Build history of the part. All positions in model axes, mm. A direction names the side the tool comes from. Give positions to 0.01 mm unless a question says otherwise; leave off trailing zeros. Order: outer loops, then holes, each group sorted by start corner. A loop starts at its lowest first (then second) coordinate and runs counter-clockwise, first axis right, second up. Notation, with made-up numbers: (17, 79) - (57, 79) arc R28 cw to (57, 105) - close; hole circle Ø10 at (-25.75, -25.5). An arc over 180 degrees is marked (long way). Answer in a Markdown table with one row per item.
```python
from build123d import *

# Parameters (mm, degrees)
BOSS_EXTRU_1_DEPTH                                = 11.6
ESQUISSE2_R                                       = 10
BOSS_EXTRU_2_DEPTH                                = 3
ENL_V_MAT_EXTRU_1_DEPTH                           = 35.026203138
ENL_V_MAT_EXTRU_1_DEPTH_BACK                      = 35.026203138
ESQUISSE3_R                                       = 1.6
ESQUISSE3_R_2                                     = 3
CHAMBRAGE_POUR_VIS_SIX_PANS_CREUX_M41_D           = 3.2
CHAMBRAGE_POUR_VIS_SIX_PANS_CREUX_M41_CBORE_D     = 6
CHAMBRAGE_POUR_VIS_SIX_PANS_CREUX_M41_CBORE_DEPTH = 8
ENL_V_MAT_EXTRU_2_DEPTH                           = 38.537081666
ENL_V_MAT_EXTRU_2_DEPTH_BACK                      = 38.537081666
CHANFREIN1_SIZE                                   = 2
CHANFREIN2_SIZE                                   = 1


with BuildPart() as part:
    # Esquisse1 → Boss.-Extru.1 (new body)
    with BuildSketch(Plane(origin=(0, 0, 0), x_dir=(1, 0, 0), z_dir=(0, 1, 0))):
        Polygon((7.5, 27.85), (-7.5, 27.85), (-7.5, 10.85), (-13, 5), (-13, -5), (-7.5, -10.85), (-7.5, -27.85), (7.5, -27.85), (7.5, -10.85), (13, -5), (13, 5), (7.5, 10.85), align=None)
    extrude(amount=BOSS_EXTRU_1_DEPTH)

    # Esquisse2 → Boss.-Extru.2 (add)
    with BuildSketch(Plane(origin=(0, 11.6, 0), x_dir=(1, 0, 0), z_dir=(0, 1, 0))):
        with Locations(Location((0, 0, 0), (0, 0, 270))):
            Circle(ESQUISSE2_R)
    extrude(amount=BOSS_EXTRU_2_DEPTH)

    # Esquisse3 → Enlèv. mat.-Extru.1 (cut, two sides: drawn at the far end of the back side and taken through both)
    with BuildSketch(Plane.XZ.offset(-ENL_V_MAT_EXTRU_1_DEPTH_BACK)):
        with Locations(Location((0, 7, 0), (0, 0, 270))):
            Circle(ESQUISSE3_R)
        with Locations(Location((7, 0, 0), (0, 0, 270))):
            Circle(ESQUISSE3_R)
        with Locations(Location((0, -7, 0), (0, 0, 270))):
            Circle(ESQUISSE3_R)
        with Locations(Location((-7, 0, 0), (0, 0, 270))):
            Circle(ESQUISSE3_R)
        with Locations(Location((0, 0, 0), (0, 0, 270))):
            Circle(ESQUISSE3_R_2)
    extrude(amount=ENL_V_MAT_EXTRU_1_DEPTH + ENL_V_MAT_EXTRU_1_DEPTH_BACK, mode=Mode.SUBTRACT)

    # Chambrage pour vis à six pans creux M41 (through all)
    with Locations(Plane(origin=(0, 0, 0), x_dir=(-1, 0, 0), z_dir=(0, -1, 0))):
        with Locations((0, 0), (0, 7), (7, 0), (0, -7), (-7, 0)):
            CounterBoreHole(CHAMBRAGE_POUR_VIS_SIX_PANS_CREUX_M41_D / 2, CHAMBRAGE_POUR_VIS_SIX_PANS_CREUX_M41_CBORE_D / 2, CHAMBRAGE_POUR_VIS_SIX_PANS_CREUX_M41_CBORE_DEPTH)

    # Esquisse6 → Enlèv. mat.-Extru.2 (cut, two sides: drawn at the far end of the back side and taken through both)
    with BuildSketch(Plane.ZY.offset(7.5).offset(-ENL_V_MAT_EXTRU_2_DEPTH_BACK)):
        Polygon((16.1, 6.810362971), (17.85, 7.820725942), (19.6, 6.810362971), (19.6, 4.789637029), (17.85, 3.779274058), (16.1, 4.789637029), align=None)
        Polygon((-17.85, 7.820725942), (-19.6, 6.810362971), (-19.6, 4.789637029), (-17.85, 3.779274058), (-16.1, 4.789637029), (-16.1, 6.810362971), align=None)
    extrude(amount=ENL_V_MAT_EXTRU_2_DEPTH + ENL_V_MAT_EXTRU_2_DEPTH_BACK, mode=Mode.SUBTRACT)

    # Chanfrein1
    chanfrein1_edges = [part.edges().sort_by_distance(p)[0] for p in [
        (0, 11.6, 27.85),
        (0, 11.6, -27.85),
    ]]
    chamfer(chanfrein1_edges, length=CHANFREIN1_SIZE)

    # Chanfrein2
    chanfrein2_edges = [part.edges().sort_by_distance(p)[0] for p in [
        (0, 14.6, -10),
    ]]
    chamfer(chanfrein2_edges, length=CHANFREIN2_SIZE)


solid = part.part
```
1. Cut at B-B on y = 10.25. Write the cut outline in (x, z).
Check result:
| item | result |
|---|---|
| outline | (-13, -5) - (-7.5, -10.85) - (-7.5, -27.2) - (7.5, -27.2) - (7.5, -10.85) - (13, -5) - (13, 5) - (7.5, 10.85) - (7.5, 27.2) - (-7.5, 27.2) - (-7.5, 10.85) - (-13, 5) - close; hole circle Ø3.2 at (-7, 0); hole circle Ø6 at (0, 0); hole circle Ø3.2 at (0, -7); hole circle Ø3.2 at (0, 7); hole circle Ø3.2 at (7, 0) |
2. Which spindle directions (+Z, -Z, +X, -X, +Y, -Y) get a long thin tool onto all of the face, cutting with end or side? Do faces 5 (the face through (0.105, 7.308, 16.963)), 6 (the face through (7.5, 4, -19)), 7 (the face through (-8.3, 8, 1.3)). Say none if no direction does.
Check result:
| item | result |
|---|---|
| face 5 | +X, -X |
| face 6 | -Z, +X, +Y, -Y |
| face 7 | -Y |
3. Cut at C-C on z = -17. Write the cut outline in (x, y), and give its area (3 significant figures).
Check result:
| item | result |
|---|---|
| outline | (-7.5, 0) - (7.5, 0) - (7.5, 4.27) - (-7.5, 4.27) - close; (-7.5, 7.33) - (7.5, 7.33) - (7.5, 11.6) - (-7.5, 11.6) - close |
| area | 128 mm² |
4. Two-plate mould, pull along Z, no slides. Class faces 1 (the face through (-10.21, 5.72, -7.97)), 2 (the face through (-7.5, 4, -19)), 3 (the face through (0.105, 4.277, -16.987)), 4 (the face through (0, 6, -19.6)): +Z half, -Z half, draft (parallel to the pull), parting line (faces both ways), or undercut.
Check result:
| item | result |
|---|---|
| face 1 | -Z half |
| face 2 | draft |
| face 3 | undercut |
| face 4 | undercut |
5. Probe line 1 (Z direction, x = 0, y = 5.75); line 2 (Z direction, x = 0.25, y = 10.5); line 3 (Z direction, x = 0, y = 4.25). List the from-to ranges inside material, lowest first.
Check result:
| item | result |
|---|---|
| line 1 | z = -27.85 to -19.6, -16.1 to -10, -4 to -3, 3 to 4, 10 to 16.1, 19.6 to 27.85 |
| line 2 | z = -26.95 to -8.58, -5.42 to -2.99, 2.99 to 5.42, 8.58 to 26.95 |
| line 3 | z = -27.85 to -18.67, -17.03 to -10, -4 to -3, 3 to 4, 10 to 17.03, 18.67 to 27.85 |
6. Drop flat-ended pins along their axis: P1, Ø1.5, axis at x = -1, z = 8.5, coming from the -Y side; P2, Ø3.5, axis at y = 5, z = 16, coming from the +X side; P3, Ø5, axis at x = 4, z = -12, coming from the +Y side. Give the stop position or say it passes through.
Check result:
| item | result |
|---|---|
| P1 | stops at y = 8 |
| P2 | stops at x = 7.5 |
| P3 | stops at y = 11.6 |
7. Cut at A-A on z = 0. Count the separate pieces of the cut face and the enclosed holes in it, and give its area (3 significant figures).
Check result:
| item | result |
|---|---|
| separate pieces | 4 |
| enclosed holes | 0 |
| area | 135 mm² |
